The model under review builds one solid part; all positions refer to its coordinate system, in mm. A direction names the side the tool comes from. Round coordinates to 2 decimals unless told otherwise and drop trailing zeros. Loops run counter-clockwise (first coordinate to the right, second up) from the corner with the lowest first, then second, coordinate; pieces in that order, holes last. Notation, with made-up numbers: M -22,-4 L -1,-4 A15 ccw -1,5 Z; hole C 35.25,-38.5 d11. An arc over 180 degrees is marked long. Return JSON: item names as keys, results as strings. Group by question number.
Q1. Draft analysis for pull direction Y (two halves, no side actions). For faces 1 (the face through (-4, 1, 10)), 2 (the face through (-0.29, 2.23, 2.96)), 3 (the face through (0, -75, 5)), 4 (the face through (0, 75, 5)), state which applies: pulls with the +Y half, pulls with the -Y half, needs draft (parallel to the pull), parting line crosses it, or undercut.
Q2. For faces 5 (the face through (2.3, -65.7, 6)), 6 (the face through (3, 1, 0)), list the 3-axis set-ups (+Z, -Z, +X, -X, +Y, -Y) from which the entire face can be reached by the end or side of a thin tool; tool diameter is ignored.
Q3. Consider section A-A (x = 0). State the section outline as (y, z) points.
Q4. Consider section C-C (z = 3.25). State the section outline as (x, y) points.
Q5. To check wall thickness, follow line 1 along Y through (x, z) = (0, 3.15); line 2 along Y through (x, z) = (0, 7.35); line 3 along X through (y, z) = (-65, 4.4). State the ranges of each line that lie inside material, in increasing order.
Q6. Clearance check with flat-ended pins moving along their axes: pin 1 Ø6 at (x, y) = (0, 65) entering from +Z; pin 2 Ø3.5 at (x, y) = (0, 0) entering from -Z. State where each tip first meets the part, or that it passes through.
Q7. Consider section B-B (y = -65). State the section outline as (x, z) points, and give its area (3 significant figures).
from build123d import *

# Parameters (mm, degrees)
CROQUIS1_W              = 12
CROQUIS1_H              = 150
CROQUIS1_R              = 2.25
SALIENTE_EXTRUIR1_DEPTH = 10
CROQUIS2_R              = 3.5
CORTAR_EXTRUIR1_DEPTH   = 4


with BuildPart() as part:
    # Croquis1 → Saliente-Extruir1 (new body)
    with BuildSketch(Plane.XY):
        Rectangle(CROQUIS1_W, CROQUIS1_H)
        with Locations((0, 65)):
            Circle(CROQUIS1_R, mode=Mode.SUBTRACT)
        Circle(CROQUIS1_R, mode=Mode.SUBTRACT)
        with Locations((0, -65)):
            Circle(CROQUIS1_R, mode=Mode.SUBTRACT)
    extrude(amount=SALIENTE_EXTRUIR1_DEPTH)

    # Croquis2 → Cortar-Extruir1 (cut)
    with BuildSketch(Plane.XY.offset(10)):
        with Locations((0, 65)):
            Circle(CROQUIS2_R)
        Circle(CROQUIS2_R)
        with Locations((0, -65)):
            Circle(CROQUIS2_R)
    extrude(amount=-CORTAR_EXTRUIR1_DEPTH, mode=Mode.SUBTRACT)


solid = part.part
Values:
{
 "1": {"face 1": "needs draft", "face 2": "undercut", "face 3": "pulls with the -Y half", "face 4": "pulls with the +Y half"},
 "2": {"face 5": "+Z", "face 6": "-Z, +X, -X, +Y, -Y"},
 "3": {"outline": "M -75,0 L -67.25,0 L -67.25,6 L -68.5,6 L -68.5,10 L -75,10 Z; M -62.75,0 L -2.25,0 L -2.25,6 L -3.5,6 L -3.5,10 L -61.5,10 L -61.5,6 L -62.75,6 Z; M 2.25,0 L 62.75,0 L 62.75,6 L 61.5,6 L 61.5,10 L 3.5,10 L 3.5,6 L 2.25,6 Z; M 67.25,0 L 75,0 L 75,10 L 68.5,10 L 68.5,6 L 67.25,6 Z"},
 "4": {"outline": "M -6,-75 L 6,-75 L 6,75 L -6,75 Z; hole C 0,-65 d4.5; hole C 0,0 d4.5; hole C 0,65 d4.5"},
 "5": {"line 1": "y = -75 to -67.25, -62.75 to -2.25, 2.25 to 62.75, 67.25 to 75", "line 2": "y = -75 to -68.5, -61.5 to -3.5, 3.5 to 61.5, 68.5 to 75", "line 3": "x = -6 to -2.25, 2.25 to 6"},
 "6": {"pin 1": "stops at z = 6", "pin 2": "passes through"},
 "7": {"outline": "M -6,0 L -2.25,0 L -2.25,6 L -3.5,6 L -3.5,10 L -6,10 Z; M 2.25,0 L 6,0 L 6,10 L 3.5,10 L 3.5,6 L 2.25,6 Z", "area": "65.0 mm2"}
}
